from build123d import *

# Parameters (mm, degrees)
PAD_DEPTH       = 31
SKETCH001_W     = 13.134895
SKETCH001_H     = 10.824528
POCKET_DEPTH    = 15
SKETCH002_W     = 13.312798
SKETCH002_H     = 10.464958
POCKET001_DEPTH = 15
FILLET_R        = 1
FILLET001_R     = 1
FILLET002_R     = 1
FILLET003_R     = 1
FILLET004_R     = 1
FILLET005_R     = 1
FILLET006_R     = 1
CHAMFER_SIZE    = 1
FILLET007_R     = 1
FILLET008_R     = 1
FILLET009_R     = 1
CHAMFER001_SIZE = 1
SKETCH003_W     = 10.93087
SKETCH003_H     = 6.35841
POCKET002_DEPTH = 16
SKETCH004_W     = 11.221859
SKETCH004_H     = 6.266699
POCKET003_DEPTH = 17
CHAMFER002_SIZE = 1
CHAMFER003_SIZE = 1


with BuildPart() as part:
    # Sketch → Pad (new body)
    with BuildSketch(Plane.XZ):
        Polygon((-32, 20), (32, 20), (32, 7), (41.5, 7), (41.5, 0), (30, 0), (30, 18), (-30, 18), (-30, 0), (-41.5, 0), (-41.5, 7), (-32, 7), align=None)
    extrude(amount=PAD_DEPTH)

    # Sketch001 (on Face13 of Pad) → Pocket (cut)
    with BuildSketch(Plane(origin=(0, 0, 0), x_dir=(1, 0, 0), z_dir=(0, 1, 0))):
        with Locations((-36.5674475, -3.587736)):
            Rectangle(SKETCH001_W, SKETCH001_H)
    extrude(amount=-POCKET_DEPTH, mode=Mode.SUBTRACT)

    # Sketch002 (on Face5 of Pocket) → Pocket001 (cut)
    with BuildSketch(Plane.XZ.offset(31)):
        with Locations((36.656399, 3.767521)):
            Rectangle(SKETCH002_W, SKETCH002_H)
    extrude(amount=-POCKET001_DEPTH, mode=Mode.SUBTRACT)

    # Fillet
    fillet_edges = [part.edges().sort_by_distance(p)[0] for p in [
        (32, -15.5, 20),
    ]]
    fillet(fillet_edges, radius=FILLET_R)

    # Fillet001
    fillet001_edges = [part.edges().sort_by_distance(p)[0] for p in [
        (-32, -15.5, 20),
    ]]
    fillet(fillet001_edges, radius=FILLET001_R)

    # Fillet002
    fillet002_edges = [part.edges().sort_by_distance(p)[0] for p in [
        (-31, -15, 9),
    ]]
    fillet(fillet002_edges, radius=FILLET002_R)

    # Fillet003
    fillet003_edges = [part.edges().sort_by_distance(p)[0] for p in [
        (-31, 0, 9),
    ]]
    fillet(fillet003_edges, radius=FILLET003_R)

    # Fillet004
    fillet004_edges = [part.edges().sort_by_distance(p)[0] for p in [
        (31, -16, 9),
    ]]
    fillet(fillet004_edges, radius=FILLET004_R)

    # Fillet005
    fillet005_edges = [part.edges().sort_by_distance(p)[0] for p in [
        (31, -31, 9),
    ]]
    fillet(fillet005_edges, radius=FILLET005_R)

    # Fillet006
    fillet006_edges = [part.edges().sort_by_distance(p)[0] for p in [
        (41.5, -8, 7),
    ]]
    fillet(fillet006_edges, radius=FILLET006_R)

    # Chamfer
    chamfer_edges = [part.edges().sort_by_distance(p)[0] for p in [
        (30, -8, 0),
    ]]
    chamfer(chamfer_edges, length=CHAMFER_SIZE)

    # Fillet007
    fillet007_edges = [part.edges().sort_by_distance(p)[0] for p in [
        (41.5, -8, 0),
    ]]
    fillet(fillet007_edges, radius=FILLET007_R)

    # Fillet008
    fillet008_edges = [part.edges().sort_by_distance(p)[0] for p in [
        (-41.5, -23, 7),
    ]]
    fillet(fillet008_edges, radius=FILLET008_R)

    # Fillet009
    fillet009_edges = [part.edges().sort_by_distance(p)[0] for p in [
        (-41.5, -23, 0),
    ]]
    fillet(fillet009_edges, radius=FILLET009_R)

    # Chamfer001
    chamfer001_edges = [part.edges().sort_by_distance(p)[0] for p in [
        (-30, -23, 0),
    ]]
    chamfer(chamfer001_edges, length=CHAMFER001_SIZE)

    # Sketch003 (on Face21 of Chamfer001) → Pocket002 (cut)
    with BuildSketch(Plane(origin=(0, 0, 0), x_dir=(1, 0, 0), z_dir=(0, 1, 0))):
        with Locations((37.465435, -5.179205)):
            Rectangle(SKETCH003_W, SKETCH003_H)
    extrude(amount=-POCKET002_DEPTH, mode=Mode.SUBTRACT)

    # Sketch004 (on Face1 of Pocket002) → Pocket003 (cut)
    with BuildSketch(Plane.XZ.offset(31)):
        with Locations((-37.6109295, 5.1333495)):
            Rectangle(SKETCH004_W, SKETCH004_H)
    extrude(amount=-POCKET003_DEPTH, mode=Mode.SUBTRACT)

    # Chamfer002
    chamfer002_edges = [part.edges().sort_by_distance(p)[0] for p in [
        (-32, -23, 2),
    ]]
    chamfer(chamfer002_edges, length=CHAMFER002_SIZE)

    # Chamfer003
    chamfer003_edges = [part.edges().sort_by_distance(p)[0] for p in [
        (32, -8, 2),
    ]]
    chamfer(chamfer003_edges, length=CHAMFER003_SIZE)


solid = part.part
The model under review builds one solid part; all positions refer to its coordinate system, in mm. A direction names the side the tool comes from. Round coordinates to 2 decimals unless told otherwise and drop trailing zeros. Loops run counter-clockwise (first coordinate to the right, second up) from the corner with the lowest first, then second, coordinate; pieces in that order, holes last. Notation, with made-up numbers: (47, 41.5) -> (104, 41.5) arc R24 ccw to (104, 68.5) -> close; hole circle Ø3 at (64.5, 37.25). An arc over 180 degrees is marked (long way). Answer as CSV lines item,"result".
1) Add section D-D on x = -15.5. Write out the cut boundary in (y, z), plus the area to 3 significant figures.
Geometry results:
outline,"(-31, 18) -> (0, 18) -> (0, 20) -> (-31, 20) -> close"
area,"62.0 mm²"
2) For P1, Ø9, axis at x = 34.5, z = 3, coming from the -Y side; P2, Ø2, axis at x = 15, y = -7, coming from the -Z side; P3, Ø1, axis at x = 33, z = 8, coming from the +Y side; P4, Ø1.5, axis at y = -26, z = 8.5, coming from the -X side, all flat-tipped, find the tip position at first contact; note any pin that passes through.
Geometry results:
P1,"stops at y = -16"
P2,"stops at z = 18"
P3,"passes through"
P4,"stops at x = -32"
3) Add section B-B on y = -5. Write out the cut boundary in (x, z), plus the area to 3 significant figures.
Geometry results:
outline,"(-32, 9) -> (-30, 9) -> (-30, 18) -> (30, 18) -> (30, 1) -> (31, 0) -> (40.5, 0) arc R1 ccw to (41.5, 1) -> (41.5, 2) -> (33, 2) -> (32, 3) -> (32, 19) arc R1 ccw to (31, 20) -> (-31, 20) arc R1 ccw to (-32, 19) -> close"
area,"200 mm²"
4) Add section C-C on z = 14.25. Write out the cut boundary in (x, y).
Geometry results:
outline,"(-32, -31) -> (-30, -31) -> (-30, 0) -> (-32, 0) -> close; (30, -31) -> (32, -31) -> (32, 0) -> (30, 0) -> close"
5) Add section A-A on z = 4. Write out the cut boundary in (x, y).
Geometry results:
outline,"(-32, -31) -> (-30, -31) -> (-30, -15) -> (-32, -15) -> close; (30, -16) -> (32, -16) -> (32, 0) -> (30, 0) -> close"
6) Tool access review of faces 1 (the face through (-37, -23, 2)), 2 (the face through (32, -15, 13)), 3 (the face through (33, -16, 1)), 4 (the face through (-33, -15, 1)), 5 (the face through (-30, -19, 12)): name each direction out of +Z, -Z, +X, -X, +Y, -Y from which nothing blocks a thin tool from reaching the whole face with its end or side.
Geometry results:
face 1,"+Z, -X, +Y, -Y"
face 2,"+Z, +X, +Y, -Y"
face 3,"-Z, +X, -Y"
face 4,"-Z, -X, +Y"
face 5,"-Z, +Y, -Y"
7) To check wall thickness, follow line 1 along X through (y, z) = (-21, 13); line 2 along Z through (x, y) = (23, -19); line 3 along X through (y, z) = (-23, 6). State the ranges of each line that lie inside material, in increasing order. Write a range as from..to.
Geometry results:
line 1,"x = -32..-30, 30..32"
line 2,"z = 18..20"
line 3,"x = -32..-30"
8) Draft analysis for pull direction X (two halves, no side actions). For faces 6 (the face through (30, -12, 11)), 7 (the face through (0, -15, 18)), 8 (the face through (-32, -15, 13)), 9 (the face through (31, -24, 9)), state which applies: pulls with the +X half, pulls with the -X half, needs draft (parallel to the pull), parting line crosses it, or undercut.
Geometry results:
face 6,"undercut"
face 7,"undercut"
face 8,"pulls with the -X half"
face 9,"needs draft"
